from build123d import *

# Parameters (mm, degrees)
F0_R     = 40.005
F0_R_2   = 8.001
F1_DEPTH = 170.688
F0_W     = 14.732
F0_H     = 14.732
F0_R_3   = 3.5941
F2_DEPTH = 9.906
F3_DEPTH = 12.6492
F4_DEPTH = 40.005
F5_R     = 5.08
F6_R     = 5.08


with BuildPart() as f1:
    # F0 (on Front) → F1 (new body)
    with BuildSketch(Plane.XZ):
        Polygon((-29.972, -29.972), (-29.972, -44.704), (-13.335, -44.704), (13.335, -44.704), (29.972, -44.704), (29.972, -29.972), (44.704, -29.972), (44.704, 29.972), (29.972, 29.972), (29.972, 44.704), (-29.972, 44.704), (-29.972, 29.972), (-44.704, 29.972), (-44.704, -29.972), align=None)
        Circle(F0_R, mode=Mode.SUBTRACT)
        Circle(F0_R)
        Circle(F0_R_2, mode=Mode.SUBTRACT)
        Circle(F0_R_2)
    extrude(amount=-F1_DEPTH)

    # F0 (on Front) → F2 (join)
    with BuildSketch(Plane.XZ):
        Polygon((-29.972, -29.972), (-29.972, -44.704), (-13.335, -44.704), (13.335, -44.704), (29.972, -44.704), (29.972, -29.972), (44.704, -29.972), (44.704, 29.972), (29.972, 29.972), (29.972, 44.704), (-29.972, 44.704), (-29.972, 29.972), (-44.704, 29.972), (-44.704, -29.972), align=None)
        Circle(F0_R, mode=Mode.SUBTRACT)
        with Locations((-37.338, 37.338)):
            Rectangle(F0_W, F0_H)
        with Locations((-35.355268, 35.355268)):
            Circle(F0_R_3, mode=Mode.SUBTRACT)
        with Locations((37.338, 37.338)):
            Rectangle(F0_W, F0_H)
        with Locations((35.355268, 35.355268)):
            Circle(F0_R_3, mode=Mode.SUBTRACT)
        with Locations((37.338, -37.338)):
            Rectangle(F0_W, F0_H)
        with Locations((35.355268, -35.355268)):
            Circle(F0_R_3, mode=Mode.SUBTRACT)
        with Locations((-37.338, -37.338)):
            Rectangle(F0_W, F0_H)
        with Locations((-35.355268, -35.355268)):
            Circle(F0_R_3, mode=Mode.SUBTRACT)
    extrude(amount=F2_DEPTH)

    # F0 (on Front) → F3 (join)
    with BuildSketch(Plane.XZ):
        Circle(F0_R)
        Circle(F0_R_2, mode=Mode.SUBTRACT)
    extrude(amount=F3_DEPTH)

    # F0 (on Front) → F4 (join)
    with BuildSketch(Plane.XZ):
        Circle(F0_R_2)
    extrude(amount=F4_DEPTH)

    # F5
    f5_edges = [f1.edges().sort_by_distance(p)[0] for p in [
        (44.704, 85.344, 29.972),
        (29.972, 85.344, 44.704),
        (44.704, 85.344, -29.972),
        (29.972, 85.344, -44.704),
        (-29.972, 85.344, -44.704),
        (-44.704, 85.344, -29.972),
        (-29.972, 85.344, 44.704),
        (-29.972, 85.344, 29.972),
        (-44.704, 85.344, 29.972),
        (-29.972, 85.344, -29.972),
        (29.972, 85.344, -29.972),
        (29.972, 85.344, 29.972),
    ]]
    fillet(f5_edges, radius=F5_R)

    # F6
    f6_edges = [f1.edges().sort_by_distance(p)[0] for p in [
        (-44.704, -4.953, 44.704),
        (-44.704, -4.953, -44.704),
        (44.704, -4.953, 44.704),
        (44.704, -4.953, -44.704),
    ]]
    fillet(f6_edges, radius=F6_R)


solid = f1.part
Verification items for the finished model (mm, model axes). A direction names the side the tool comes from. Coordinates: 2 decimals unless noted, no trailing zeros. Write each loop counter-clockwise with the first axis right and the second up, starting at its lowest first coordinate (ties: lowest second). Pieces come first, ordered by that corner, then holes. Notation, with made-up numbers: M -8.5,42 L 26.5,42 A25 ccw 26.5,76 Z; hole C -19.5,-21 d3. An arc over 180 degrees is marked long. Use CSV: the item, a comma, the result in double quotes.
Q1. Go/stop test with flat-tipped pins: P1, Ø5, axis at y = 99.5, z = -36.5, coming from the +X side; P2, Ø2.5, axis at y = 66, z = 38, coming from the +X side; P3, Ø3.5, axis at x = -38.5, y = 85, coming from the -Z side. Record where each tip stops, or that it passes through.
Computed values:
P1,"x = 30.08"
P2,"x = 29.97"
P3,"z = -29.97"
Q2. Section check D-D, the plane x = 20.5. Enter the section's corners in (y, z).
Computed values:
outline,"M -12.65,-34.35 L -9.91,-34.35 L -9.91,-44.7 L 170.69,-44.7 L 170.69,44.7 L -9.91,44.7 L -9.91,34.35 L -12.65,34.35 Z"
Q3. Section check C-C, the plane x = 0. Enter the section's corners in (y, z) (3 decimals).
Computed values:
outline,"M -40.005,-8.001 L -12.649,-8.001 L -12.649,-40.005 L -9.906,-40.005 L -9.906,-44.704 L 170.688,-44.704 L 170.688,44.704 L -9.906,44.704 L -9.906,40.005 L -12.649,40.005 L -12.649,8.001 L -40.005,8.001 Z"
Q4. Set-up check for faces 4 (the flat face through (-1, 82, -44.704)), 5 (the cylindrical face through (-28.4, 86.5, -43.3)), 6 (the flat face through (37, 0, -39)), 7 (the cylindrical face through (28.4, 86.5, 43.3)): record each of +Z, -Z, +X, -X, +Y, -Y from which the full face is reachable in a straight line by a thin tool's end or side.
Computed values:
face 4,"-Z, +X, -X, +Y, -Y"
face 5,"-Z, -X, +Y"
face 6,"-Z, +X, +Y"
face 7,"+Z, +X, +Y"
Q5. Section check B-B, the plane y = 40.5. Enter the section's corners in (x, z), and give its area (3 significant figures).
Computed values:
outline,"M -44.7,-24.89 A5.08 ccw -39.62,-29.97 L -35.05,-29.97 A5.08 cw -29.97,-35.05 L -29.97,-39.62 A5.08 ccw -24.89,-44.7 L 24.89,-44.7 A5.08 ccw 29.97,-39.62 L 29.97,-35.05 A5.08 cw 35.05,-29.97 L 39.62,-29.97 A5.08 ccw 44.7,-24.89 L 44.7,24.89 A5.08 ccw 39.62,29.97 L 35.05,29.97 A5.08 cw 29.97,35.05 L 29.97,39.62 A5.08 ccw 24.89,44.7 L -24.89,44.7 A5.08 ccw -29.97,39.62 L -29.97,35.05 A5.08 cw -35.05,29.97 L -39.62,29.97 A5.08 ccw -44.7,24.89 Z"
area,"7,100 mm²"
Q6. Mould release check, pull along Z, two halves, no side actions. Record for faces 1 (the cylindrical face through (-43.3, 86.5, 28.4)), 2 (the cylindrical face through (28.4, 86.5, -43.3)), 3 (the cylindrical face through (38.783, -4.884, 36.435)): pulls with the +Z half, pulls with the -Z half, needs draft (parallel to the pull), parting line crosses it, or undercut.
Computed values:
face 1,"pulls with the +Z half"
face 2,"pulls with the -Z half"
face 3,"undercut"
Q7. Thickness scan on line 1 along Y through (x, z) = (24.5, 17); line 2 along Y through (x, z) = (38, 38.5); line 3 along Z through (x, y) = (35, 142.5). Record the ranges inside material, lowest first. Write a range as [from, to].
Computed values:
line 1,"[-12.65, 170.69]"
line 2,"[-9.91, 0]"
line 3,"[-29.97, 29.97]"
Q8. Section check A-A, the plane z = 0. Enter the section's corners in (x, y) (3 decimals), and give its area (3 significant figures).
Computed values:
outline,"M -44.704,-9.906 L -40.005,-9.906 L -40.005,-12.649 L -8.001,-12.649 L -8.001,-40.005 L 8.001,-40.005 L 8.001,-12.649 L 40.005,-12.649 L 40.005,-9.906 L 44.704,-9.906 L 44.704,170.688 L -44.704,170.688 Z"
area,"16,800 mm²"
